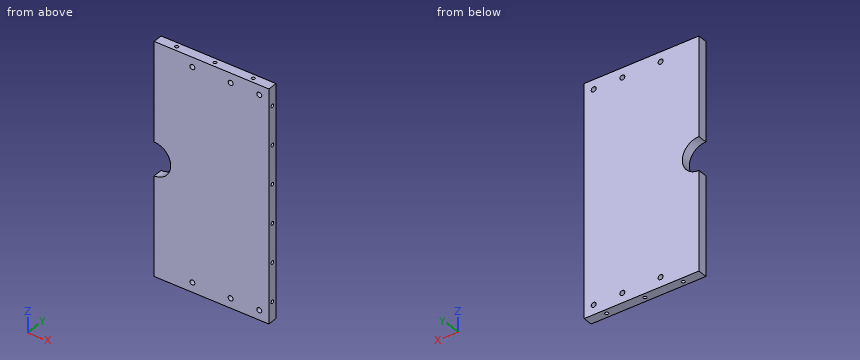
from build123d import *

# Parameters (mm, degrees)
SKETCH1_R           = 1.63195
BOSS_EXTRUDE1_DEPTH = 6.35
LPATTERN1_COUNT     = 6
LPATTERN1_PITCH     = 25.4
LPATTERN2_COUNT     = 3
LPATTERN2_PITCH     = 25.4


with BuildPart() as part:
    # Sketch1 → Boss-Extrude1 (new body)
    with BuildSketch(Plane(origin=(0, 0, 0), x_dir=(1, 0, 0), z_dir=(0, 1, 0))):
        with BuildLine():
            Line((0, -11), (0, -76.2))
            Line((0, -76.2), (76.2, -76.2))
            Line((76.2, -76.2), (76.2, 76.2))
            Line((76.2, 76.2), (0, 76.2))
            Line((0, 76.2), (0, 11))
            ThreePointArc((0, 11), (11, 0), (0, -11))
        make_face()
        with Locations((69.85, 69.85)):
            Circle(SKETCH1_R, mode=Mode.SUBTRACT)
        with Locations((69.85, -69.85)):
            Circle(SKETCH1_R, mode=Mode.SUBTRACT)
        with Locations((50.8, 69.85)):
            Circle(SKETCH1_R, mode=Mode.SUBTRACT)
        with Locations((25.4, 69.85)):
            Circle(SKETCH1_R, mode=Mode.SUBTRACT)
        with Locations((50.8, -69.85)):
            Circle(SKETCH1_R, mode=Mode.SUBTRACT)
        with Locations((25.4, -69.85)):
            Circle(SKETCH1_R, mode=Mode.SUBTRACT)
    extrude(amount=BOSS_EXTRUDE1_DEPTH)

    # Sketch2 → #4-40 Tapped Hole1 (revolve, cut)
    with BuildSketch(Plane(origin=(76.2, 3.175, 63.5), x_dir=(0, 0, -1), z_dir=(0, 1, 0))):
        Polygon((0, 0), (0, 8.279152758), (1.1303, 7.6), (1.1303, 0), align=None)
    f_4_40_tapped_hole1 = revolve(axis=Axis((82.55, 3.175, 63.5), (-1, 0, 0)), mode=Mode.SUBTRACT)

    # LPattern1: #4-40 Tapped Hole1 ×6
    with Locations(*[(0, 0, -i * LPATTERN1_PITCH) for i in range(1, LPATTERN1_COUNT)]):
        add(f_4_40_tapped_hole1, mode=Mode.SUBTRACT)

    # Sketch3 → #4-40 Tapped Hole2 (revolve, cut)
    with BuildSketch(Plane(origin=(63.5, 3.175, 76.2), x_dir=(0, -1, 0), z_dir=(1, 0, 0))):
        Polygon((0, 0), (0, 8.279152758), (1.1303, 7.6), (1.1303, 0), align=None)
    f_4_40_tapped_hole2 = revolve(axis=Axis((63.5, 3.175, 82.55), (0, 0, -1)), mode=Mode.SUBTRACT)

    # LPattern2: #4-40 Tapped Hole2 ×3
    with Locations(*[(-i * LPATTERN2_PITCH, 0, 0) for i in range(1, LPATTERN2_COUNT)]):
        add(f_4_40_tapped_hole2, mode=Mode.SUBTRACT)

    # Mirror1: #4-40 Tapped Hole2 across plane
    add(f_4_40_tapped_hole2.mirror(Plane.XY), mode=Mode.SUBTRACT)

    # Mirror1 copy 1 sketch → Mirror1 copy 1 (revolve, cut)
    with BuildSketch(Plane(origin=(38.1, 3.175, -76.2), x_dir=(0, -1, 0), z_dir=(1, 0, 0))):
        Polygon((0, 0), (0, -8.279152758), (1.1303, -7.6), (1.1303, 0), align=None)
    revolve(axis=Axis((38.1, 3.175, -82.55), (0, 0, -1)), mode=Mode.SUBTRACT)

    # Mirror1 copy 2 sketch → Mirror1 copy 2 (revolve, cut)
    with BuildSketch(Plane(origin=(12.7, 3.175, -76.2), x_dir=(0, -1, 0), z_dir=(1, 0, 0))):
        Polygon((0, 0), (0, -8.279152758), (1.1303, -7.6), (1.1303, 0), align=None)
    revolve(axis=Axis((12.7, 3.175, -82.55), (0, 0, -1)), mode=Mode.SUBTRACT)


solid = part.part
Work out the finished part from the listing and answer in its coordinate system (mm). Give positions to 0.01 mm unless a question says otherwise; leave off trailing zeros. Order: outer loops, then holes, each group sorted by start corner. A loop starts at its lowest first (then second) coordinate and runs counter-clockwise, first axis right, second up. Notation, with made-up numbers: (51, -14) -> (75, -14) arc R18 cw to (75, 1) -> close; hole circle Ø1 at (38.5, 28.5). An arc over 180 degrees is marked (long way). One line per item, written item: value.
Item 1: Straight lines are drawn through the part: probe 1 along Z at (x, y) = (25.4, 3.75); probe 2 along Y at (x, z) = (70.75, -63.5); probe 3 along X at (y, z) = (3.5, 3). For each, find the intervals that lie inside material, in ascending order.
Answer sheet:
probe 1: -76.2 to -71.48, -68.22 to 68.22, 71.48 to 76.2
probe 2: 0 to 2.04, 4.31 to 6.35
probe 3: 10.58 to 76.2
Item 2: Find section A-A, the plane x = 25.4. Give the vertices of the cut face in (y, z).
Answer sheet:
outline: (0, -76.2) -> (6.35, -76.2) -> (6.35, -71.48) -> (0, -71.48) -> close; (0, -68.22) -> (6.35, -68.22) -> (6.35, 68.22) -> (0, 68.22) -> close; (0, 71.48) -> (6.35, 71.48) -> (6.35, 76.2) -> (0, 76.2) -> close
Item 3: Find section B-B, the plane x = 9. Give the vertices of the cut face in (y, z).
Answer sheet:
outline: (0, -76.2) -> (6.35, -76.2) -> (6.35, -6.32) -> (0, -6.32) -> close; (0, 6.32) -> (6.35, 6.32) -> (6.35, 76.2) -> (0, 76.2) -> close
Item 4: Find section C-C, the plane z = 0. Give the vertices of the cut face in (x, y).
Answer sheet:
outline: (11, 0) -> (76.2, 0) -> (76.2, 6.35) -> (11, 6.35) -> close
Item 5: Flat-ended cylindrical pins translate along their axes: P1, Ø3.5, axis at x = 63.5, y = 3.175, coming from the -Z side; P2, Ø2, axis at x = 12.7, y = 3.175, coming from the +Z side; P3, Ø2, axis at y = 2, z = -4.5, coming from the -X side. Find the tip coordinate at first contact, or state that the pin passes through.
Answer sheet:
P1: z = -76.2
P2: z = 68.52
P3: x = 9.53
